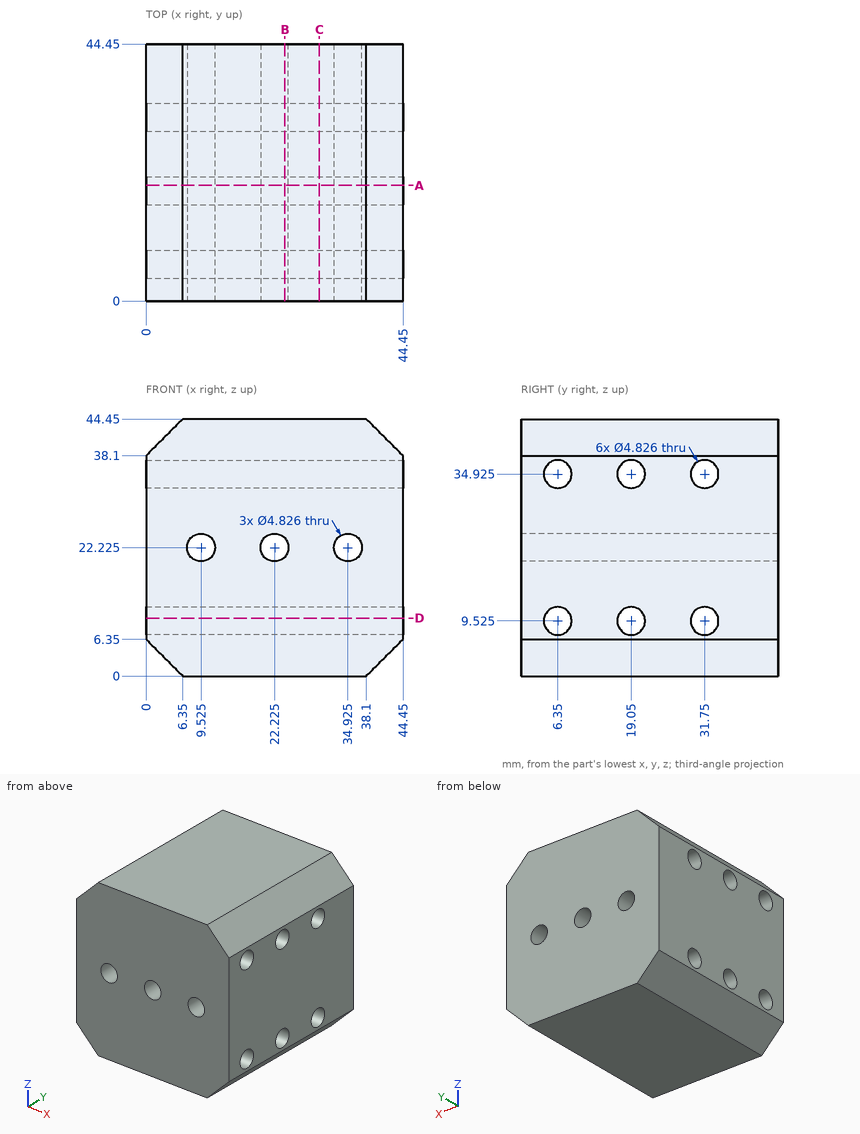
Source: three-view drawing plus pictorial views. Frame: mm from the lowest corner of the part. Give positions to 0.01 mm unless a question says otherwise; leave off trailing zeros. Order: outer loops, then holes, each group sorted by start corner. A loop starts at its lowest first (then second) coordinate and runs counter-clockwise, first axis right, second up. Notation, with made-up numbers: M -12.5,58 L 34.5,58 A16 ccw 34.5,81 Z; hole C -3,66.5 d4. An arc over 180 degrees is marked long. One line per question, with ' | ' between items.
1) Ray query, L1, parallel to Y at x = 22, z = 9.5; L2, parallel to X at y = 12, z = 22; L3, parallel to Z at x = 16, y = 18. Return the intervals inside material, ascending.
Filled in:
L1: y = 0 to 3.94, 8.76 to 16.64, 21.46 to 29.34, 34.16 to 44.45 | L2: x = 0 to 7.12, 11.93 to 19.82, 24.63 to 32.52, 37.33 to 44.45 | L3: z = 0 to 7.35, 11.7 to 32.75, 37.1 to 44.45
2) Section C-C on x = 30. Output: boundary loops of the cut face in (y, z) (3 decimals).
Filled in:
outline: M 0,0 L 44.45,0 L 44.45,44.45 L 0,44.45 Z; hole C 6.35,9.525 d4.826; hole C 6.35,34.925 d4.826; hole C 19.05,9.525 d4.826; hole C 19.05,34.925 d4.826; hole C 31.75,9.525 d4.826; hole C 31.75,34.925 d4.826
3) Section A-A on y = 20. Output: boundary loops of the cut face in (x, z) (3 decimals).
Filled in:
outline: M 0,6.35 L 6.35,0 L 38.1,0 L 44.45,6.35 L 44.45,7.307 L 0,7.307 Z; M 0,11.743 L 44.45,11.743 L 44.45,32.707 L 0,32.707 Z; M 0,37.143 L 44.45,37.143 L 44.45,38.1 L 38.1,44.45 L 6.35,44.45 L 0,38.1 Z; hole C 9.525,22.225 d4.826; hole C 22.225,22.225 d4.826; hole C 34.925,22.225 d4.826
4) Contact query for a flat-ended pin moving along its axis: P1, Ø4.5, axis at y = 31.75, z = 34.925, coming from the +X side. Output: stop coordinate, or through.
Filled in:
P1: passes through
5) Section B-B on x = 24. Output: boundary loops of the cut face in (y, z) (3 decimals), and give its area (3 significant figures).
Filled in:
outline: M 0,0 L 44.45,0 L 44.45,20.59 L 0,20.59 Z; M 0,23.86 L 44.45,23.86 L 44.45,44.45 L 0,44.45 Z; hole C 6.35,9.525 d4.826; hole C 6.35,34.925 d4.826; hole C 19.05,9.525 d4.826; hole C 19.05,34.925 d4.826; hole C 31.75,9.525 d4.826; hole C 31.75,34.925 d4.826 | area: 1,720 mm2
6) Section D-D on z = 10. Output: boundary loops of the cut face in (x, y), and give its area (3 significant figures).
Filled in:
outline: M 0,0 L 44.45,0 L 44.45,3.98 L 0,3.98 Z; M 0,8.72 L 44.45,8.72 L 44.45,16.68 L 0,16.68 Z; M 0,21.42 L 44.45,21.42 L 44.45,29.38 L 0,29.38 Z; M 0,34.12 L 44.45,34.12 L 44.45,44.45 L 0,44.45 Z | area: 1,340 mm2
